Could you check a few things on this drawing? It's one solid part, dimensions in mm from its lowest x, y, z. Give positions to 0.01 mm unless a question says otherwise; leave off trailing zeros. Loops run counter-clockwise (first coordinate to the right, second up) from the corner with the lowest first, then second, coordinate; pieces in that order, holes last.
1. I need wall thicknesses on line 1 along Y through (x, z) = (4, 6); line 2 along Y through (x, z) = (1.5, 6.25); line 3 along X through (y, z) = (40.5, 5). Which ranges of each line are inside material? Lowest first, please.
2. Imagine slicing it at B-B (x = 1.5). List the corners of the cut face in (y, z) for me.
3. Imagine slicing it at C-C (y = 40.5). List the corners of the cut face in (x, z) for me, plus the area to 3 significant figures.
4. Imagine slicing it at A-A (z = 6). List the corners of the cut face in (x, y) for me, plus the area to 3 significant figures.
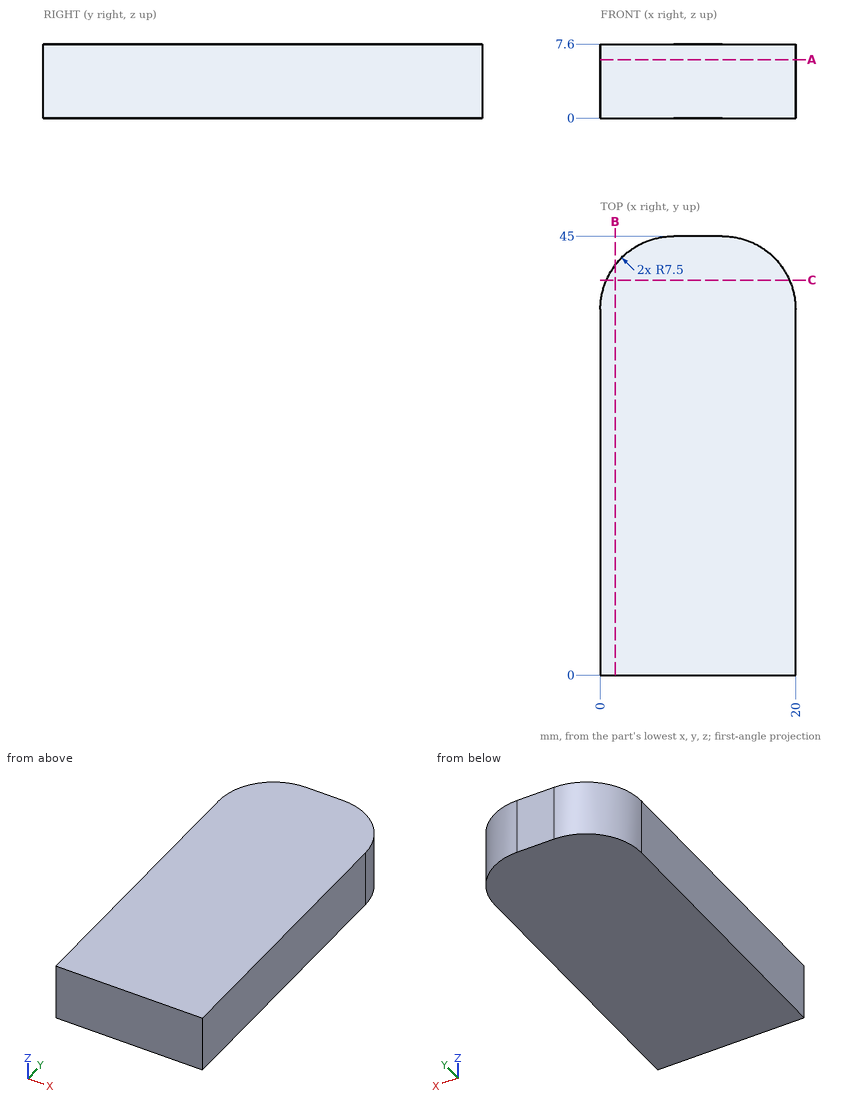
Derived:
1. line 1: y = 0 to 44.13
1. line 2: y = 0 to 42
1. line 3: x = 0.63 to 19.37
2. outline: (0, 0) - (42, 0) - (42, 7.6) - (0, 7.6) - close
3. outline: (0.63, 0) - (19.37, 0) - (19.37, 7.6) - (0.63, 7.6) - close
3. area: 142 mm2
4. outline: (0, 0) - (20, 0) - (20, 37.5) arc R7.5 ccw to (12.5, 45) - (7.5, 45) arc R7.5 ccw to (0, 37.5) - close
4. area: 876 mm2
